Part model, mm, in its own coordinate system. A direction names the side the tool comes from. Give positions to 0.01 mm unless a question says otherwise; leave off trailing zeros. Order: outer loops, then holes, each group sorted by start corner. A loop starts at its lowest first (then second) coordinate and runs counter-clockwise, first axis right, second up. Notation, with made-up numbers: M 9,45.25 L 67,45.25 A34 ccw 67,84.25 Z; hole C 2,81.25 d8. An arc over 180 degrees is marked long. Return JSON: item names as keys, results as strings.
Autodesk Inventor part; units mm, degrees
ref_plane "Work Plane1" through (5.0748, 0, 6.0527) normal (0.6448, -0.4106, 0.6448) x (0.5371, 0.8435, 0)
ref_plane "YZ Plane" through (0, 0, 0) normal (1, 0, 0) x (0, 1, 0)
ref_plane "XZ Plane" through (0, 0, 0) normal (0, 1, 0) x (-1, 0, 0)
sketch "Sketch1" plane through (0, 0, 0) normal (0, 0, 1) x (1, 0, 0)
  line L0 (-0.9779, 24.003) -> (1.7526, 24.003)
  line L1 (1.7526, 24.003) -> (1.7526, 22.5552)
  line L2 (1.7526, 22.5552) -> (4.2926, 22.5552)
  line L3 (4.2926, 22.5552) -> (9.5377, 17.0688)
  line L4 (9.5377, 17.0688) -> (9.5377, 4.3434)
  line L5 (9.5377, 4.3434) -> (7.5819, 0)
  line L6 (7.5819, 0) -> (0, 0)
  line L7 (-0.9779, -11.5824) -> (-0.9779, 24.003)
  line L8 (-0.9779, -8.6887) -> (-0.9779, -11.5824)
  line L9 (-0.9779, -11.5824) -> (0, -11.5824)
  line L10 (0, -11.5824) -> (0, 0)
  dimension "d0" = 24.003
  dimension "d1" = 10.5156
  dimension "d2" = 22.5552
  dimension "d3" = 17.0688
  dimension "d4" = 4.3434
  dimension "d5" = 2.7305
  dimension "d6" = 11.5824
  dimension "d7" = 0.9779
  dimension "d9" = 5.2705
  dimension "d10" = 8.5598
revolve "Revolution1" add sketch "Sketch1" angle 360 about axis through (-0.9779, -11.5824, 0) along (0, 1, 0)
sketch "Sketch2" plane through (-0.9779, 0, 0) normal (0, -1, 0) x (1, 0, 0)
  circle A0 centre (0, 0) radius 0.9779
  circle A1 centre (0, 0) radius 8.5598
  line L0 (6.1849, 3.0099) -> (13.589, 3.0099)
  line L1 (16.5989, 0) -> (16.5989, 0)
  line L2 (13.589, -3.0099) -> (6.1849, -3.0099)
  line L3 (3.0099, -6.1849) -> (3.0099, -13.589)
  line L4 (0, -16.5989) -> (0, -16.5989)
  line L5 (-3.0099, -13.589) -> (-3.0099, -6.1849)
  line L6 (-6.1849, -3.0099) -> (-13.589, -3.0099)
  line L7 (-16.5989, 0) -> (-16.5989, 0)
  line L8 (-13.589, 3.0099) -> (-6.1849, 3.0099)
  line L9 (-3.0099, 6.1849) -> (-3.0099, 13.589)
  line L10 (0, 16.5989) -> (0, 16.5989)
  line L11 (3.0099, 13.589) -> (3.0099, 6.1849)
  arc A2 (-6.1849, 3.0099) -> (-3.0099, 6.1849) centre (-6.1849, 6.1849) ccw
  arc A3 (3.0099, 6.1849) -> (6.1849, 3.0099) centre (6.1849, 6.1849) ccw
  arc A4 (6.1849, -3.0099) -> (3.0099, -6.1849) centre (6.1849, -6.1849) ccw
  arc A5 (-3.0099, -6.1849) -> (-6.1849, -3.0099) centre (-6.1849, -6.1849) ccw
  arc A6 (16.5989, 0) -> (13.589, 3.0099) centre (13.589, 0) ccw
  arc A7 (13.589, -3.0099) -> (16.5989, 0) centre (13.589, 0) ccw
  arc A8 (-13.589, 3.0099) -> (-16.5989, 0) centre (-13.589, 0) ccw
  arc A9 (-16.5989, 0) -> (-13.589, -3.0099) centre (-13.589, 0) ccw
  arc A10 (-3.0099, -13.589) -> (0, -16.5989) centre (0, -13.589) ccw
  arc A11 (0, -16.5989) -> (3.0099, -13.589) centre (0, -13.589) ccw
  arc A12 (0, 16.5989) -> (-3.0099, 13.589) centre (0, 13.589) ccw
  arc A13 (3.0099, 13.589) -> (0, 16.5989) centre (0, 13.589) ccw
  circle A14 centre (0, 0) radius 4.1021
  circle A15 centre (0, 13.589) radius 1.4986
  circle A16 centre (13.589, 0) radius 1.4986
  circle A17 centre (-13.589, 0) radius 1.4986
  circle A18 centre (0, -13.589) radius 1.4986
  point P0 (0.9779, 0)
  dimension "d15" = 6.0198
  dimension "d16" = 3.175
  dimension "d17" = 3.0099
  dimension "d18" = 13.589
  dimension "d19" = 13.589
  dimension "d20" = 13.589
  dimension "d21" = 8.2042
  dimension "d22" = 2.9972
extrude "Extrusion1" add sketch "Sketch2" along normal blind 1.0922 contours A1 L2 A4 L3 L5 A5 L6 L8 A2 L9 L11 A3 L0 | A1 L0 A6 A7 L2 | A1 L9 A12 A13 L11 | L3 A11 A10 L5 A1 | A1 L6 A9 A8 L8
ref_plane "Work Plane1" through (5.0748, 0, 6.0527) normal (0.6448, -0.4106, 0.6448) x (0.5371, 0.8435, 0)
sketch "Sketch3" plane through (5.0748, 0, 6.0527) normal (0.6448, -0.4106, 0.6448) x (0.5371, 0.8435, 0)
  line L0 (3.28, 3.0554) -> (4.5151, 0.3869)
  line L1 (2.3848, 2.6411) -> (3.62, -0.0274)
  arc A0 (3.28, 3.0554) -> (2.3848, 2.6411) centre (2.8324, 2.8483) ccw
  arc A1 (3.62, -0.0274) -> (4.5151, 0.3869) centre (4.0675, 0.1797) ccw
  point P0 (-2.7259, -1.8667)
extrude "Extrusion2" add sketch "Sketch3" along normal blind 1.5875 and the other way blind 0.254
sketch "Sketch4" plane through (6.0983, -0.6518, 7.0762) normal (0.6448, -0.4106, 0.6448) x (0.5438, -0.3463, -0.7644)
  arc A0 (0.0274, 3.62) -> (-0.3869, 4.5151) centre (-0.1797, 4.0675) ccw
  arc A1 (-3.0554, 3.28) -> (-2.6411, 2.3848) centre (-2.8483, 2.8324) ccw
  line L0 (0.0274, 3.62) -> (-2.6411, 2.3848)
  circle A2 centre (-2.4072, 3.0365) radius 0.3811
  circle A3 centre (-1.514, 3.45) radius 0.3811
  circle A4 centre (-0.6208, 3.8634) radius 0.3811
  line L1 (-2.8483, 2.8324) -> (-0.1797, 4.0675) construction
  line L2 (-2.4072, 3.0365) -> (-1.514, 3.45)
  line L3 (-1.514, 3.45) -> (-0.6208, 3.8634)
  line L4 (-2.4072, 3.0365) -> (-2.8483, 2.8324) construction
  line L5 (-2.4072, 3.0365) -> (-2.8483, 2.8324) construction
  line L6 (-0.6208, 3.8634) -> (-0.1797, 4.0675) construction
  point P0 (1.8667, -2.7259)
extrude "Extrusion3" cut sketch "Sketch4" against normal blind 0.254
sketch "Sketch5" plane through (7.6722, 2.9262, 7.387) normal (0.6448, -0.4106, 0.6448) x (0.7071, 0, -0.7071)
  circle A0 centre (0, 0) radius 0.3811 construction
sketch "Sketch6" plane through (6.9643, 2.8868, 8.0698) normal (0.6448, -0.4106, 0.6448) x (0.7071, 0, -0.7071)
  circle A0 centre (0, 0) radius 0.3811 construction
sketch "Sketch7" plane through (6.2565, 2.8475, 8.7525) normal (0.6448, -0.4106, 0.6448) x (0.7071, 0, -0.7071)
  circle A0 centre (0, 0) radius 0.3811 construction
properties part number "Thrust_Motor"
Q1. Two-plate mould, pull along Y, no slides. Class faces 4 (the flat face through (-1, 24.003, 0)), 5 (the conical face through (7.3, 0.27, -2.61)), 6 (the flat face through (-10.9, -0.5, 3.01)): +Y half, -Y half, draft (parallel to the pull), parting line (faces both ways), or undercut.
Established:
{"face 4": "+Y half", "face 5": "undercut", "face 6": "draft"}
Q2. Band-saw the part on B-B (z = 13). Give the cut face in (x, y).
Established:
{"outline": "M -3.99,-1.09 L -2.36,-1.09 L -2.36,0 L -3.99,0 Z; M 0.4,-1.09 L 2.03,-1.09 L 2.03,0 L 0.4,0 Z"}
Q3. 3-axis set-ups, long thin cutter, end or side, ignore diameter. For faces 1 (the flat face through (6.431, 2.686, 7.535)), 2 (the flat face through (-6, 0, 5)), 3 (the flat face through (6.686, 3.585, 7.851)): which of +Z, -Z, +X, -X, +Y, -Y reach the whole face in a straight line?
Established:
{"face 1": "-Y", "face 2": "+Z, -X, -Y", "face 3": "+Z, +X"}
Q4. Band-saw the part on C-C (z = -11.5). Give the cut face in (x, y), then the cut area to 3 significant figures.
Established:
{"outline": "M -3.99,-1.09 L 2.03,-1.09 L 2.03,0 L -3.99,0 Z", "area": "6.57 mm²"}
Q5. Probe line 1 along Y through (x, z) = (-1.5, 2.5); line 2 along Y through (x, z) = (0.5, -11); line 3 along Z through (x, y) = (4, 20). List the from-to ranges inside material, lowest first.
Established:
{"line 1": "y = 0 to 24", "line 2": "y = -1.09 to 0", "line 3": "z = -5.89 to 5.89"}
Q6. Pin check, flat tips, straight feed: pin 1 (8 mm diameter, centred on y = 4, z = 9.5, fed in from -X); pin 2 (6.5 mm diameter, centred on x = -0.5, z = 12.5, fed in from +Y); pin 3 (5 mm diameter, centred on x = -14.57, z = 0, fed in from -Y); pin 4 (16.5 mm diameter, centred on x = 3, z = 6.5, fed in from -Y). Stop position of each tip, or through.
Established:
{"pin 1": "stops at x = -9.93", "pin 2": "stops at y = 18.38", "pin 3": "stops at y = -1.09", "pin 4": "stops at y = -11.58"}
Q7. Band-saw the part on A-A (z = 0). Give the number of separate pieces and of enclosed holes in the cut face, then the cut area to 3 significant figures.
Established:
{"separate pieces": "3", "enclosed holes": "0", "area": "488 mm²"}
